Read the model definition and answer for the solid it produces. Units are mm, in the model's axes. Face numbers are marked on the shaded views. A direction names the side the tool comes from. Round coordinates to 2 decimals unless told otherwise and drop trailing zeros. Order: outer loops, then holes, each group sorted by start corner. A loop starts at its lowest first (then second) coordinate and runs counter-clockwise, first axis right, second up. Notation, with made-up numbers: (-29.5, 7) - (-12.5, 7) arc R11 cw to (-12.5, 26) - close; hole circle Ø1 at (11, -19.5). An arc over 180 degrees is marked (long way). Answer as a JSON object with one key per item and string values. Group by question number.
Q1. The mould has two halves that part along X. Classify the marked faces 1, 2 and 3: pulls with the +X half, pulls with the -X half, needs draft (parallel to the pull), parting line crosses it, or undercut.
Q2. A cutting plane is placed at C-C on y = 0. Determine the outline of the cut face in (x, z).
Q3. A cutting plane is placed at A-A on z = 34. Determine the outline of the cut face in (x, y), and give its area (3 significant figures).
Q4. A cutting plane is placed at B-B on x = 0. Determine the outline of the cut face in (y, z), and give its area (3 significant figures).
Q5. A cutting plane is placed at D-D on y = 10.5. Determine the outline of the cut face in (x, z).
Q6. Consider line 1 (Z direction, x = 23, y = 3); line 2 (Y direction, x = 0, z = 16); line 3 (Y direction, x = 1.5, z = 22). Determine where each line is inside the solid, lowest interval first.
Q7. A tool of negligible diameter and unlimited length cuts with its end or side. For the marked faces 4 and 5, from which of +Z, -Z, +X, -X, +Y, -Y can it reach the whole face along a straight path? Write none if from no direction.
Q8. Given pin 1 Ø4 at (y, z) = (10, 22.5) entering from +X; pin 2 Ø2.5 at (x, y) = (-0.5, 10) entering from +Z; pin 3 Ø9.5 at (x, y) = (-0.5, -10.5) entering from +Z; pin 4 Ø12 at (x, z) = (-15, 28) entering from +Y, each flat-ended and moving along its own axis, determine where each tip first touches the part or whether it passes through.
```python
from build123d import *

# Parameters (mm, degrees)
EXTRUDE_1_DEPTH          = 10
SKETCH_3_R               = 5
CUT_EXTRUDE_1_DEPTH      = 10
SKETCH_4_R               = 16
EXTRUDE_2_DEPTH          = 33
SKETCH_5_R               = 9
CUT_EXTRUDE_2_DEPTH      = 89
CUT_EXTRUDE_3_DEPTH      = 89
CUT_EXTRUDE_3_DEPTH_BACK = 89
SKETCH_6_W               = 10
SKETCH_6_H               = 12


with BuildPart() as part:
    # 草图1 → 凸台-拉伸1 (new body)
    with BuildSketch(Plane.XY):
        with BuildLine():
            Line((-36.911764706, 8.515963028), (-6.470588235, 18.924362285))
            ThreePointArc((-6.470588235, 18.924362285), (0, 20), (6.470588235, 18.924362285))
            Line((6.470588235, 18.924362285), (36.911764706, 8.515963028))
            ThreePointArc((36.911764706, 8.515963028), (43, 0), (36.911764706, -8.515963028))
            Line((36.911764706, -8.515963028), (6.470588235, -18.924362285))
            ThreePointArc((6.470588235, -18.924362285), (0, -20), (-6.470588235, -18.924362285))
            Line((-6.470588235, -18.924362285), (-36.911764706, -8.515963028))
            ThreePointArc((-36.911764706, -8.515963028), (-43, 0), (-36.911764706, 8.515963028))
        make_face()
    extrude(amount=EXTRUDE_1_DEPTH)

    # 草图3 → 切除-拉伸1 (cut)
    with BuildSketch(Plane.XY):
        with Locations((-34, 0)):
            Circle(SKETCH_3_R)
        with Locations((34, 0)):
            Circle(SKETCH_3_R)
    extrude(amount=CUT_EXTRUDE_1_DEPTH, mode=Mode.SUBTRACT)

    # 草图4 → 凸台-拉伸2 (add)
    with BuildSketch(Plane.XY.offset(10)):
        Circle(SKETCH_4_R)
    extrude(amount=EXTRUDE_2_DEPTH)

    # 草图5 → 切除-拉伸2 (cut)
    with BuildSketch(Plane.XY.offset(43)):
        Circle(SKETCH_5_R)
    extrude(amount=-CUT_EXTRUDE_2_DEPTH, mode=Mode.SUBTRACT)

    # 草图6 → 切除-拉伸3 (cut, two sides: drawn at the far end of the back side and taken through both)
    with BuildSketch(Plane(origin=(0, 0, 0), x_dir=(1, 0, 0), z_dir=(0, 1, 0)).offset(-CUT_EXTRUDE_3_DEPTH_BACK)):
        with Locations((0, -37)):
            Rectangle(SKETCH_6_W, SKETCH_6_H)
    extrude(amount=CUT_EXTRUDE_3_DEPTH + CUT_EXTRUDE_3_DEPTH_BACK, mode=Mode.SUBTRACT)


solid = part.part
```
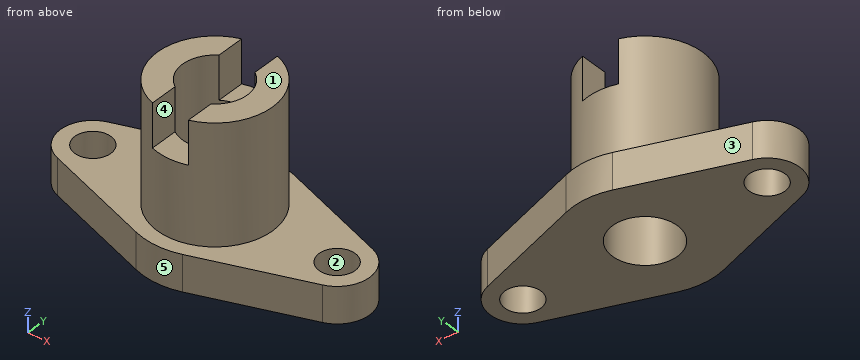
Result set:
{
 "1": {"face 1": "needs draft", "face 2": "undercut", "face 3": "pulls with the -X half"},
 "2": {"outline": "(-43, 0) - (-39, 0) - (-39, 10) - (-43, 10) - close; (-29, 0) - (-9, 0) - (-9, 43) - (-16, 43) - (-16, 10) - (-29, 10) - close; (9, 0) - (29, 0) - (29, 10) - (16, 10) - (16, 43) - (9, 43) - close; (39, 0) - (43, 0) - (43, 10) - (39, 10) - close"},
 "3": {"outline": "(-5, -15.2) - (-5, -7.48) arc R9 cw to (-5, 7.48) - (-5, 15.2) arc R16 ccw to start; (5, -15.2) arc R16 ccw to (5, 15.2) - (5, 7.48) arc R9 cw to (5, -7.48) - close", "area": "405 mm²"},
 "4": {"outline": "(-20, 0) - (-9, 0) - (-9, 31) - (-16, 31) - (-16, 10) - (-20, 10) - close; (9, 0) - (20, 0) - (20, 10) - (16, 10) - (16, 31) - (9, 31) - close", "area": "514 mm²"},
 "5": {"outline": "(-31.11, 0) - (31.11, 0) - (31.11, 10) - (12.07, 10) - (12.07, 43) - (5, 43) - (5, 31) - (-5, 31) - (-5, 43) - (-12.07, 43) - (-12.07, 10) - (-31.11, 10) - close"},
 "6": {"line 1": "z = 0 to 10", "line 2": "y = -16 to -9, 9 to 16", "line 3": "y = -15.93 to -8.87, 8.87 to 15.93"},
 "7": {"face 4": "+Z, +Y, -Y", "face 5": "+Z, -Z, -Y"},
 "8": {"pin 1": "stops at x = 13.86", "pin 2": "stops at z = 31", "pin 3": "stops at z = 43", "pin 4": "stops at y = 13.23"}
}
